Could you check a few things on this model? Use its own coordinates, in mm. A direction names the side the tool comes from. Round coordinates to 2 decimals unless told otherwise and drop trailing zeros. Loops run counter-clockwise (first coordinate to the right, second up) from the corner with the lowest first, then second, coordinate; pieces in that order, holes last. Notation, with made-up numbers: (-28, -2.75) -> (18, -2.75) arc R16 cw to (18, 24.25) -> close; hole circle Ø2 at (-34.75, 65.5). An arc over 180 degrees is marked (long way). One line per item, written item: value.
```python
from build123d import *

# Parameters (mm, degrees)
BOSS_EXTRU_1_DEPTH = 5
BOSS_EXTRU_2_DEPTH = 5


with BuildPart() as part:
    # Esquisse1 → Boss.-Extru.1 (new body)
    with BuildSketch(Plane.XY):
        Polygon((-16, -12), (-16, -5), (16, -5), (16, -12), (35, -12), (35, -17), (40, -17), (40, -5), (25, -5), (25, 0), (-25, 0), (-25, -5), (-40, -5), (-40, -17), (-35, -17), (-35, -12), align=None)
    extrude(amount=BOSS_EXTRU_1_DEPTH)

    # Esquisse2 → Boss.-Extru.2 (add)
    with BuildSketch(Plane.XY.offset(5)):
        with BuildLine():
            Line((-16, -10), (-16, -3.900376605))
            Line((-16, -3.900376605), (16, -3.900376605))
            Line((16, -3.900376605), (16, -10))
            ThreePointArc((16, -10), (14.535533906, -6.464466094), (11, -5))
            Line((11, -5), (-11, -5))
            ThreePointArc((-11, -5), (-14.535533906, -6.464466094), (-16, -10))
        make_face()
    extrude(amount=-BOSS_EXTRU_2_DEPTH)


solid = part.part
```
Item 1: For faces 1 (the face through (25, -3, 2)), 2 (the face through (0.6, -4.6, 5)), 3 (the face through (15, -7, 3)), 4 (the face through (-25, -2, 2)), which set-ups out of +Z, -Z, +X, -X, +Y, -Y let a thin tool reach every point of the face, with its end or its side?
Output:
face 1: +Z, -Z, +X, +Y
face 2: +Z, +X, -X, +Y, -Y
face 3: +Z, -Z, -Y
face 4: +Z, -Z, -X, +Y
Item 2: If we section it at D-D on y = -1.5: List the corners of the cut face in (x, z) for me, plus the area to 3 significant figures.
Output:
outline: (-25, 0) -> (25, 0) -> (25, 5) -> (-25, 5) -> close
area: 250 mm²
Item 3: If we section it at C-C on x = 22: List the corners of the cut face in (y, z) for me, plus the area to 3 significant figures.
Output:
outline: (-12, 0) -> (0, 0) -> (0, 5) -> (-12, 5) -> close
area: 60.0 mm²
Item 4: If we section it at A-A on y = -7: List the corners of the cut face in (x, z) for me.
Output:
outline: (-40, 0) -> (-15, 0) -> (-15, 5) -> (-40, 5) -> close; (15, 0) -> (40, 0) -> (40, 5) -> (15, 5) -> close
Item 5: If we section it at B-B on z = 1.5: List the corners of the cut face in (x, y) for me, plus the area to 3 significant figures.
Output:
outline: (-40, -17) -> (-35, -17) -> (-35, -12) -> (-16, -12) -> (-16, -10) arc R5 cw to (-11, -5) -> (11, -5) arc R5 cw to (16, -10) -> (16, -12) -> (35, -12) -> (35, -17) -> (40, -17) -> (40, -5) -> (25, -5) -> (25, 0) -> (-25, 0) -> (-25, -5) -> (-40, -5) -> close
area: 647 mm²
Item 6: If we mould it in two halves opening along X, with no side actions, what happens to faces 5 (the face through (35, -14, 2)), 6 (the face through (33, -5, 2)), 7 (the face through (-40, -11, 2))? For each: released by +X, released by -X, zero draft, split by the parting line, or undercut.
Output:
face 5: undercut
face 6: zero draft
face 7: released by -X
Item 7: I need wall thicknesses on line 1 (X direction, y = -15, z = 0.4); line 2 (X direction, y = -10.5, z = 2.5); line 3 (Y direction, x = -6, z = 3.3). Which ranges of each line are inside material? Lowest first, please. Write a range as from..to.
Output:
line 1: x = -40..-35, 35..40
line 2: x = -40..-16, 16..40
line 3: y = -5..0
Item 8: Will these pins go through, and if not, where does the flat tip stop? pin 1 Ø3 at (y, z) = (-3, 3.5) entering from -X; pin 2 Ø10 at (x, y) = (-27.5, -9.5) entering from -Z; pin 3 Ø1.5 at (x, z) = (27.5, 3.5) entering from -Y; pin 4 Ø2.5 at (x, z) = (-30.5, 1.5) entering from +Y.
Output:
pin 1: stops at x = -25
pin 2: stops at z = 0
pin 3: stops at y = -12
pin 4: stops at y = -5
